Geometry check sheet. Reference: the model listing, model coordinates, mm. Coordinates: 2 decimals unless noted, no trailing zeros. Loops run counter-clockwise (first coordinate to the right, second up) from the corner with the lowest first, then second, coordinate; pieces in that order, holes last. Notation, with made-up numbers: M 73.25,56.25 L 79.25,56.25 A29 ccw 79.25,85.25 Z; hole C -4.75,-39.5 d10. An arc over 180 degrees is marked long. Use CSV: the item, a comma, the result in double quotes.
```python
from build123d import *

# Parameters (mm, degrees)
F0_W     = 165.1
F0_H     = 101.6
F1_DEPTH = 6.35
F2_R     = 2.5527
F3_DEPTH = 25.4
F4_R     = 14.2875
F5_DEPTH = 25.4


with BuildPart() as f1:
    # F0 (on Front) → F1 (new body)
    with BuildSketch(Plane.XZ):
        with Locations((-151.574861, 50.8)):
            Rectangle(F0_W, F0_H)
    extrude(amount=F1_DEPTH)

    # F2 (on face) → F3 (cut)
    with BuildSketch(Plane.XZ.offset(6.35)):
        with Locations((-107.124861, 12.7)):
            Circle(F2_R)
        with Locations((-81.724861, 12.7)):
            Circle(F2_R)
        with Locations((-107.124861, 88.9)):
            Circle(F2_R)
        with Locations((-81.724861, 88.9)):
            Circle(F2_R)
    extrude(amount=-F3_DEPTH, mode=Mode.SUBTRACT)

    # F4 (on face) → F5 (cut)
    with BuildSketch(Plane.XZ.offset(6.35)):
        with Locations((-201.859877, 22.078976)):
            Circle(F4_R)
    extrude(amount=-F5_DEPTH, mode=Mode.SUBTRACT)


solid = f1.part
```
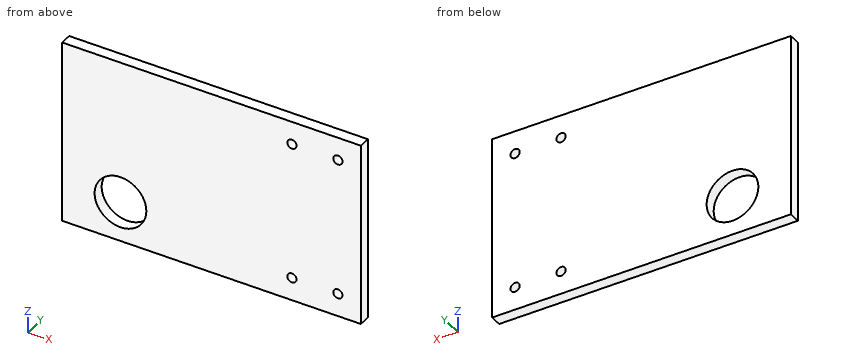
1. Thickness scan on line 1 (Z direction, x = -193, y = -5.75); line 2 (X direction, y = -4.25, z = 27); line 3 (X direction, y = -2, z = 32). Record the ranges inside material, lowest first. Write a range as [from, to].
The answers:
line 1,"[0, 10.87], [33.29, 101.6]"
line 2,"[-234.12, -215.27], [-188.45, -69.02]"
line 3,"[-234.12, -212.14], [-191.58, -69.02]"
2. Section check C-C, the plane y = -1.5. Record the cut outline in (x, z) (1 decimal), plus the area to 3 significant figures.
The answers:
outline,"M -234.1,0 L -69,0 L -69,101.6 L -234.1,101.6 Z; hole C -201.9,22.1 d28.6; hole C -107.1,12.7 d5.1; hole C -107.1,88.9 d5.1; hole C -81.7,12.7 d5.1; hole C -81.7,88.9 d5.1"
area,"16,100 mm^2"
3. Gauge pin test, flat ends, axial feed: P1, Ø23, axis at x = -201.86, z = 22.08, coming from the +Y side; P2, Ø1, axis at x = -198, y = -1.5, coming from the -Z side. Record the tip position at first contact, or that the pin passes through.
The answers:
P1,"through"
P2,"z = 0"
4. Section check A-A, the plane z = 12.7. Record the cut outline in (x, y), plus the area to 3 significant figures.
The answers:
outline,"M -234.12,-6.35 L -212.64,-6.35 L -212.64,0 L -234.12,0 Z; M -191.08,-6.35 L -109.68,-6.35 L -109.68,0 L -191.08,0 Z; M -104.57,-6.35 L -84.28,-6.35 L -84.28,0 L -104.57,0 Z; M -79.17,-6.35 L -69.02,-6.35 L -69.02,0 L -79.17,0 Z"
area,"847 mm^2"
5. Section check D-D, the plane z = 27. Record the cut outline in (x, y), plus the area to 3 significant figures.
The answers:
outline,"M -234.12,-6.35 L -215.27,-6.35 L -215.27,0 L -234.12,0 Z; M -188.45,-6.35 L -69.02,-6.35 L -69.02,0 L -188.45,0 Z"
area,"878 mm^2"
6. Section check B-B, the plane z = 88.9. Record the cut outline in (x, y).
The answers:
outline,"M -234.12,-6.35 L -109.68,-6.35 L -109.68,0 L -234.12,0 Z; M -104.57,-6.35 L -84.28,-6.35 L -84.28,0 L -104.57,0 Z; M -79.17,-6.35 L -69.02,-6.35 L -69.02,0 L -79.17,0 Z"
